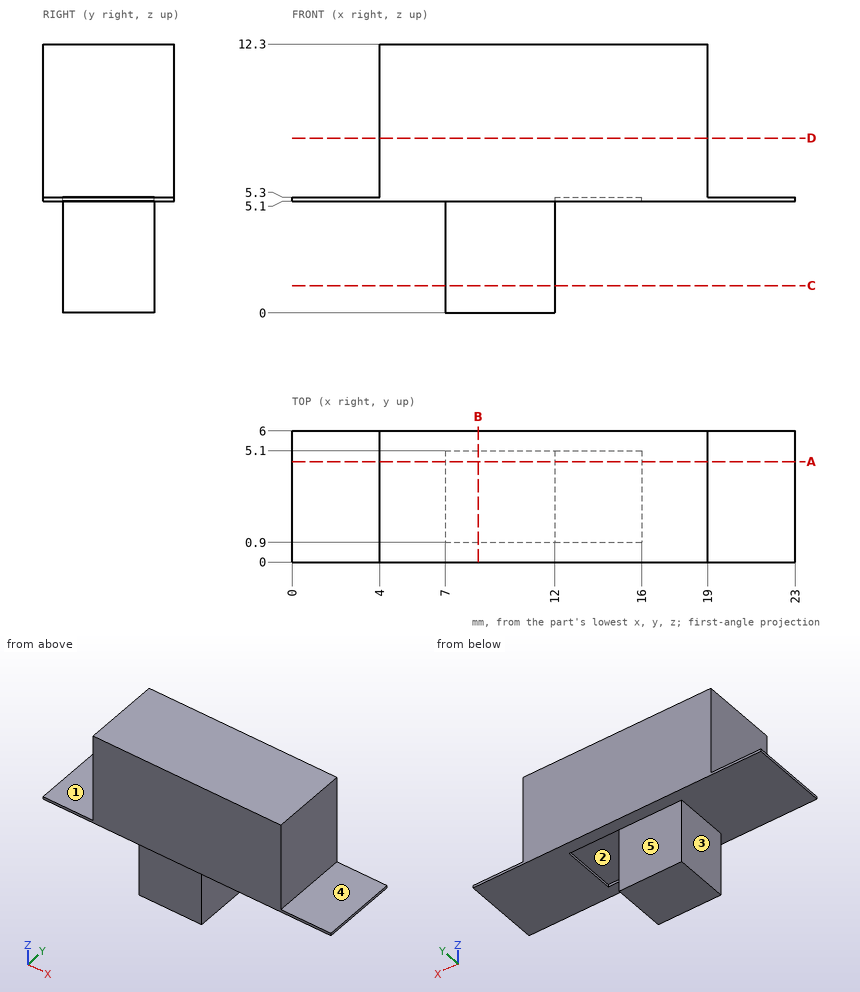
Source: three-view drawing plus pictorial views. Frame: mm from the lowest corner of the part. A direction names the side the tool comes from. Give positions to 0.01 mm unless a question says otherwise; leave off trailing zeros. Order: outer loops, then holes, each group sorted by start corner. A loop starts at its lowest first (then second) coordinate and runs counter-clockwise, first axis right, second up. Notation, with made-up numbers: M 75,33 L 92,33 A6 cw 92,40 Z; hole C 26,-23 d6. An arc over 180 degrees is marked long. Return JSON: item names as keys, results as strings.
Item 1: Cut plane B-B (x = 8.5). Return loops of the section in (y, z).
Solutions:
{"outline": "M 0,5.1 L 0.9,5.1 L 0.9,0 L 5.1,0 L 5.1,5.1 L 6,5.1 L 6,12.3 L 0,12.3 Z"}
Item 2: Cut plane C-C (z = 1.25). Return loops of the section in (x, y), then the cut area to 3 significant figures.
Solutions:
{"outline": "M 7,0.9 L 12,0.9 L 12,5.1 L 7,5.1 Z", "area": "21.0 mm^2"}
Item 3: First-contact query: P1, Ø4, axis at x = 9.5, z = 1.5, coming from the -Y side; P2, Ø1, axis at x = 16, y = 3.5, coming from the -Z side; P3, Ø3.5, axis at y = 3, z = 2, coming from the -X side; P4, Ø1.5, axis at x = 13.5, z = 3, coming from the -Y side. Flat tips, straight axial feed; report the tip coordinate or a pass-through.
Solutions:
{"P1": "y = 0.9", "P2": "z = 5.1", "P3": "x = 7", "P4": "through"}
Item 4: Cut plane D-D (z = 8). Return loops of the section in (x, y).
Solutions:
{"outline": "M 4,0 L 19,0 L 19,6 L 4,6 Z"}
Item 5: Cut plane A-A (y = 4.6). Return loops of the section in (x, z).
Solutions:
{"outline": "M 0,5.1 L 7,5.1 L 7,0 L 12,0 L 12,5.3 L 16,5.3 L 16,5.1 L 23,5.1 L 23,5.3 L 19,5.3 L 19,12.3 L 4,12.3 L 4,5.3 L 0,5.3 Z"}
Item 6: Ray query, probe 1 along X at (y, z) = (2.25, 2.5); probe 2 along Z at (x, y) = (19.75, 1.1); probe 3 along Z at (x, y) = (15.25, 5.05). Return the intervals inside material, ascending.
Solutions:
{"probe 1": "7 to 12", "probe 2": "5.1 to 5.3", "probe 3": "5.3 to 12.3"}
Item 7: Access query for the marked faces 1, 2, 3, 4 and 5. Directions: +Z, -Z, +X, -X, +Y, -Y. A direction counts if a zero-diameter tool reaches every point of the face in a straight line with its end or side. Return the directions, or none.
Solutions:
{"face 1": "+Z, -X, +Y, -Y", "face 2": "-Z", "face 3": "-Z, -X, +Y, -Y", "face 4": "+Z, +X, +Y, -Y", "face 5": "-Z, +X, -X, +Y"}
